from build123d import *

# Parameters (mm, degrees)
SKETCH1_R           = 11.05
BOSS_EXTRUDE1_DEPTH = 7.4
SKETCH3_R           = 0.83
BOSS_EXTRUDE2_DEPTH = 10.69


with BuildPart() as part:
    # Sketch1 → Boss-Extrude1 (new body)
    with BuildSketch(Plane(origin=(0, 0, 0), x_dir=(1, 0, 0), z_dir=(0, 1, 0))):
        with Locations(Location((0, 0, 0), (0, 0, 270))):
            Circle(SKETCH1_R)
    extrude(amount=BOSS_EXTRUDE1_DEPTH)

    # Sketch2 → Revolve1 (revolve)
    with BuildSketch(Plane(origin=(0, 0, 0), x_dir=(0, 0, -1), z_dir=(1, 0, 0))):
        with BuildLine():
            Line((0, 0), (0, -9.525))
            ThreePointArc((0, -9.525), (6.735192091, -6.735192091), (9.525, 0))
            Line((9.525, 0), (0, 0))
        make_face()
    revolve(axis=Axis((0, 0, 0), (0, 1, 0)))

    # Sketch3 → Boss-Extrude2 (add)
    with BuildSketch(Plane(origin=(0, 7.4, 0), x_dir=(1, 0, 0), z_dir=(0, 1, 0))):
        with Locations(Location((7.625, 0, 0), (0, 0, 270))):
            Circle(SKETCH3_R)
    boss_extrude2 = extrude(amount=BOSS_EXTRUDE2_DEPTH)

    # Mirror1: Boss-Extrude2 across plane
    add(boss_extrude2.mirror(Plane(origin=(0, 0, 0), x_dir=(0, 0, 1), z_dir=(1, 0, 0))))


solid = part.part
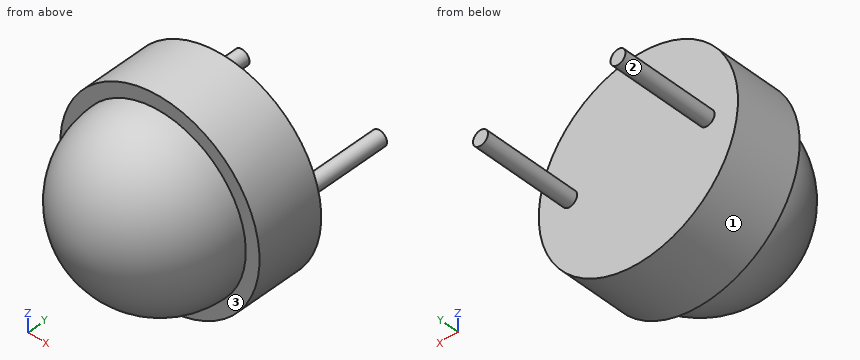
The listing builds one solid part. Answer for the finished solid, in the listing's coordinates (mm). Face numbers are marked on the shaded views. Coordinates: 2 decimals unless noted, no trailing zeros. Loops run counter-clockwise (first coordinate to the right, second up) from the corner with the lowest first, then second, coordinate; pieces in that order, holes last. Notation, with made-up numbers: (-18, 16.25) -> (0, 16.25) arc R19 cw to (0, 51.25) -> close; hole circle Ø9 at (65, -37). An arc over 180 degrees is marked (long way). Answer in a Markdown table with one row per item. Add a question column.
1. The part is cut by section D-D, the plane y = 15. Write down the section's boundary in (x, z) (3 decimals), then the cut area to 3 significant figures.
2. The part is cut by section A-A, the plane x = 0. Write down the section's boundary in (y, z) (3 decimals), then the cut area to 3 significant figures.
3. Flat-ended cylindrical pins translate along their axes: P1, Ø6, axis at y = 10.5, z = 3, coming from the -X side (3 decimals); P2, Ø1, axis at x = 0.5, z = -4, coming from the +Y side; P3, Ø1, axis at y = -4, z = 7, coming from the +X side. Find the tip coordinate at first contact, or state that the pin passes through.
4. The part is cut by section B-B, the plane y = 4.75. Write down the section's boundary in (x, z), then the cut area to 3 significant figures.
5. Determine the mould class of the marked faces 1, 2 and 3 for opening direction X: +X half, -X half, draft (parallel to the pull), parting line (faces both ways), or undercut.
6. Consider line 1 (Y direction, x = -8.75, z = -5.25); line 2 (Z direction, x = 5, y = 3.75); line 3 (X direction, y = -3.5, z = -2.25). Determine where each line is inside the solid, lowest interval first. Write a range as [from, to].
7. The part is cut by section C-C, the plane z = 7.25. Write down the section's boundary in (x, y).
Answer below:
| question | item | result |
|---|---|---|
| 1 | outline | circle Ø1.66 at (-7.625, 0); circle Ø1.66 at (7.625, 0) |
| 1 | area | 4.33 mm2 |
| 2 | outline | (0, -11.05) -> (7.4, -11.05) -> (7.4, 11.05) -> (0, 11.05) -> (0, 9.525) arc R9.525 ccw to (0, -9.525) -> close |
| 2 | area | 306 mm2 |
| 3 | P1 | x = -8.455 |
| 3 | P2 | y = 7.4 |
| 3 | P3 | x = 5.79 |
| 4 | outline | circle Ø22.1 at (0, 0) |
| 4 | area | 384 mm2 |
| 5 | face 1 | parting line |
| 5 | face 2 | undercut |
| 5 | face 3 | draft |
| 6 | line 1 | [0, 7.4] |
| 6 | line 2 | [-9.85, 9.85] |
| 6 | line 3 | [-8.57, 8.57] |
| 7 | outline | (-8.34, 0) -> (-6.18, 0) arc R6.18 ccw to (6.18, 0) -> (8.34, 0) -> (8.34, 7.4) -> (-8.34, 7.4) -> close |
